Can you work these out from the model? Positions are in its coordinate system, mm. A direction names the side the tool comes from. Give positions to 0.01 mm unless a question says otherwise; leave off trailing zeros. Order: outer loops, then holes, each group sorted by start corner. A loop starts at its lowest first (then second) coordinate and runs counter-clockwise, first axis right, second up.
Item 1: I'm going to push flat-ended pins straight in: pin 1 Ø8 at (x, z) = (74.5, 8.5) entering from -Y; pin 2 Ø10 at (y, z) = (32, 2.5) entering from +X; pin 3 Ø3 at (x, y) = (67.5, -24) entering from -Z. Where does each tip first touch, or does it pass through?
Item 2: If I drill on line 1 along Y through (x, z) = (21, 26.5); line 2 along X through (y, z) = (14.5, 10); line 3 along Y through (x, z) = (107, 23), over which ranges is the centre line in solid material (lowest first)?
Item 3: I want a section at C-C, the plane x = 26. Write out the boundary of the cut face in (y, z), then the cut area to 4 significant figures.
Item 4: If we mould it in two halves opening along Y, with no side actions, what happens to faces 5 (the cylindrical face through (108.04, -52.1, -2.14)), 6 (the flat face through (56, 1, 2.5)), 7 (the cylindrical face through (107.96, 52.1, 41.14))? For each: +Y half, -Y half, draft (parallel to the pull), parting line (faces both ways), or undercut.
Item 5: I want a section at A-A, the plane z = 8. Write out the boundary of the cut face in (x, y).
Item 6: I want a section at D-D, the plane y = -12.5. Write out the boundary of the cut face in (x, z), then the cut area to 4 significant figures.
Item 7: Which directions (+Z, -Z, +X, -X, +Y, -Y) give clear straight access to the entire face, cutting with the end or side of a thin tool? Please do faces 1 (the flat face through (108.5, -1, 20)), 2 (the cylindrical face through (107.96, 52.1, -2.14)), 3 (the flat face through (2, 0, 36)), 4 (the flat face through (2.5, -1, 19)).
Item 8: I want a section at B-B, the plane y = 0. Write out the boundary of the cut face in (x, z).
```python
from build123d import *

# Parameters (mm, degrees)
F0_W        = 105
F0_H        = 98
F1_DEPTH    = 36
F2_DEPTH    = 42
F3_DEPTH    = 3
F4_T        = 2.5
F4_T3_DEPTH = 41
F4_T5_DEPTH = 103
F5_R        = 3
F6_R        = 4
F7_DEPTH    = 3
F8_R        = 6
F9_DEPTH    = 4.7


# Not quite as in the source:
# - a shell that OpenCascade refuses in one call is made with other operations: the cavity is built on its own and cut out


with BuildPart() as f1:
    # F0 (on Top) → F1 (new body)
    with BuildSketch(Plane.XY):
        with Locations((52.5, 0)):
            Rectangle(F0_W, F0_H)
    extrude(amount=F1_DEPTH)

    # F0 (on Top) → F2 (join)
    with BuildSketch(Plane.XY):
        Polygon((105, 53), (105, 49), (105, -49), (105, -53), (111, -53), (111, 53), align=None)
    extrude(amount=F2_DEPTH)

    # F0 (on Top) → F3 (join)
    with BuildSketch(Plane.XY):
        Polygon((105, 53), (105, 49), (105, -49), (105, -53), (111, -53), (111, 53), align=None)
    extrude(amount=-F3_DEPTH)

    # F4: shell of thickness 2.5, made by hand


with BuildPart() as f4_core1:
    # F4_t2: copy of F1
    add(f1.part)

    # the walls: a layer under each face that stays
    f4_faces = [f4_core1.faces().sort_by_distance(p)[0] for p in [
        (105, 45.4285714286, 38.7857142857),
        (108, 0, 42),
        (111, 0, 19.5),
        (108, 53, 19.5),
        (108, 0, -3),
        (108, -53, 19.5),
        (0, 0, 18),
        (52.5, -49, 18),
        (52.5, 0, 0),
        (52.5, 49, 18),
    ]]
    thicken(f4_faces, amount=-F4_T, mode=Mode.SUBTRACT)

    # F4_s4 → F4_t3 (cut)
    with BuildSketch(Plane.XY.offset(-2.5)):
        Polygon((104.975, 49.025), (107.5, 49), (107.5, 46.5), (105, 46.5), align=None)
        Polygon((104.975, -49.025), (107.5, -49), (107.5, -46.5), (105, -46.5), align=None)
    extrude(amount=F4_T3_DEPTH, mode=Mode.SUBTRACT)

    # F4_s6 → F4_t5 (cut)
    with BuildSketch(Plane.XZ.offset(-51.5)):
        Polygon((104.975, -0.025), (107.5, 0), (107.5, 2.5), (105, 2.5), align=None)
    extrude(amount=F4_T5_DEPTH, mode=Mode.SUBTRACT)


with BuildPart() as f1_1:
    add(f1.part)

    # what is left inside the walls is the cavity
    f4_cavity = [f4_core1.part.solids().sort_by_distance(p)[0] for p in [
        (55, -15.5, 35.975),
    ]]
    add(f4_cavity, mode=Mode.SUBTRACT)

    # F5
    f5_edges = [f1_1.edges().sort_by_distance(p)[0] for p in [
        (108, -53, 42),
        (108, 53, 42),
        (108, 53, -3),
        (108, -53, -3),
    ]]
    fillet(f5_edges, radius=F5_R)

    # F6 (on face) → F7 (join)
    with BuildSketch(Plane.YZ.offset(111)):
        with Locations((0, 20.9335461259)):
            Circle(F6_R)
    extrude(amount=F7_DEPTH)

    # F8 (on face) → F9 (join)
    with BuildSketch(Plane.YZ.offset(114)):
        with Locations((0, 20.9335461259)):
            Circle(F8_R)
    extrude(amount=F9_DEPTH)


solid = f1_1.part
```
Results list:
1. pin 1: stops at y = -49
1. pin 2: stops at x = 111
1. pin 3: stops at z = 0
2. line 1: y = -49 to -46.5, 46.5 to 49
2. line 2: x = 0 to 2.5, 108.5 to 111
2. line 3: y = -53 to -46.5, 46.5 to 53
3. outline: (-49, 0) - (49, 0) - (49, 36) - (46.5, 36) - (46.5, 2.5) - (-46.5, 2.5) - (-46.5, 36) - (-49, 36) - close
3. area: 412.5 mm2
4. face 5: -Y half
4. face 6: undercut
4. face 7: +Y half
5. outline: (0, -49) - (105, -49) - (105, -53) - (111, -53) - (111, 53) - (105, 53) - (105, 49) - (0, 49) - close; hole (2.5, -46.5) - (107.5, -46.5) - (107.5, -50.5) - (108.5, -50.5) - (108.5, 50.5) - (107.5, 50.5) - (107.5, 46.5) - (2.5, 46.5) - close
6. outline: (0, 0) - (105, 0) - (105, -3) - (111, -3) - (111, 42) - (105, 42) - (105, 36) - (107.5, 36) - (107.5, 39.5) - (108.5, 39.5) - (108.5, -0.5) - (107.5, -0.5) - (107.5, 2.5) - (2.5, 2.5) - (2.5, 36) - (0, 36) - close
6. area: 492.5 mm2
7. face 1: none
7. face 2: -Z, +X, -X, +Y
7. face 3: +Z, -X, +Y, -Y
7. face 4: +Z
8. outline: (0, 0) - (105, 0) - (105, -3) - (111, -3) - (111, 16.93) - (114, 16.93) - (114, 14.93) - (118.7, 14.93) - (118.7, 26.93) - (114, 26.93) - (114, 24.93) - (111, 24.93) - (111, 42) - (105, 42) - (105, 36) - (107.5, 36) - (107.5, 39.5) - (108.5, 39.5) - (108.5, -0.5) - (107.5, -0.5) - (107.5, 2.5) - (2.5, 2.5) - (2.5, 36) - (0, 36) - close
